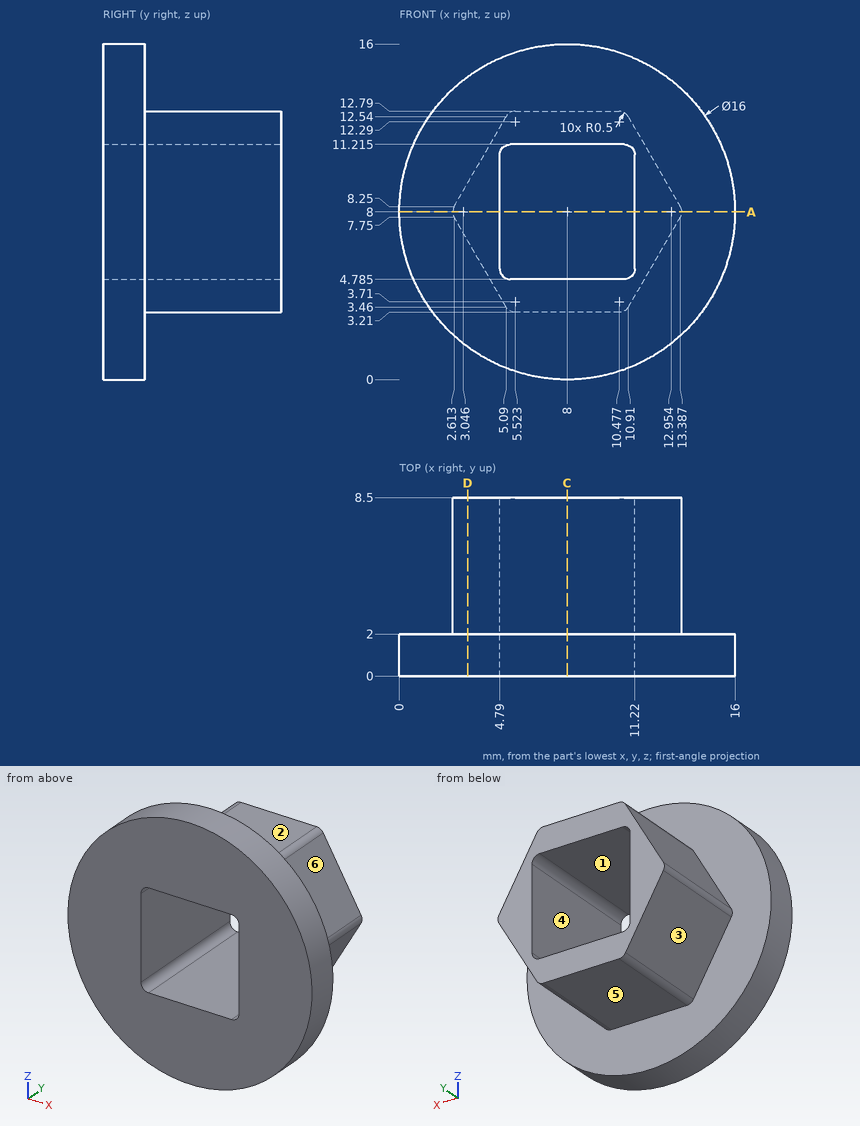
Source: three-view drawing plus pictorial views. Frame: mm from the lowest corner of the part. A direction names the side the tool comes from. Give positions to 0.01 mm unless a question says otherwise; leave off trailing zeros. Write each loop counter-clockwise with the first axis right and the second up, starting at its lowest first coordinate (ties: lowest second). Pieces come first, ordered by that corner, then holes.
(1) Cut plane D-D, the plane x = 3.25. Return loops of the section in (y, z).
(2) Cut plane A-A, the plane z = 8. Return loops of the section in (x, y).
(3) Mould query, pull axis X, two halves, no side actions, for the marked faces 4, 5 and 6. Classes: released by +X, released by -X, zero draft, split by the parting line, or undercut.
(4) Access query for the marked faces 1, 2 and 3. Directions: +Z, -Z, +X, -X, +Y, -Y. A direction counts if a zero-diameter tool reaches every point of the face in a straight line with its end or side. Return the directions, or none.
(5) First-contact query: P1, Ø1.5, axis at x = 6, y = 7, coming from the +Z side; P2, Ø3, axis at x = 13.5, y = 6, coming from the -Z side; P3, Ø1, axis at x = 9, y = 1, coming from the +Z side. Flat tips, straight axial feed; report the tip coordinate or a pass-through.
(6) Ray query, line 1 (Z direction, x = 7.25, y = 6.75) (1 decimal); line 2 (Y direction, x = 13.5, z = 5); line 3 (Z direction, x = 5, y = 5) (1 decimal). Return the intervals inside material, ascending.
(7) Cut plane C-C, the plane x = 8. Return loops of the section in (y, z) (1 decimal).
Values follow:
1. outline: (0, 1.56) - (2, 1.56) - (2, 6.65) - (8.5, 6.65) - (8.5, 9.35) - (2, 9.35) - (2, 14.44) - (0, 14.44) - close
2. outline: (0, 0) - (4.79, 0) - (4.79, 8.5) - (2.55, 8.5) - (2.55, 2) - (0, 2) - close; (11.22, 0) - (16, 0) - (16, 2) - (13.45, 2) - (13.45, 8.5) - (11.22, 8.5) - close
3. face 4: undercut
3. face 5: zero draft
3. face 6: released by +X
4. face 1: +Y, -Y
4. face 2: +Z, +X, -X, +Y
4. face 3: -Z, -X, +Y
5. P1: stops at z = 12.79
5. P2: stops at z = 5.35
5. P3: stops at z = 15.98
6. line 1: z = 3.2 to 4.8, 11.2 to 12.8
6. line 2: y = 0 to 2
6. line 3: z = 3.6 to 4.9, 11.1 to 12.4
7. outline: (0, 0) - (2, 0) - (2, 3.2) - (8.5, 3.2) - (8.5, 4.8) - (0, 4.8) - close; (0, 11.2) - (8.5, 11.2) - (8.5, 12.8) - (2, 12.8) - (2, 16) - (0, 16) - close
